Design review of the part built by this model. Coordinates are the model's own, in mm. Face numbers are marked on the shaded views. A direction names the side the tool comes from. Give positions to 0.01 mm unless a question says otherwise; leave off trailing zeros. Order: outer loops, then holes, each group sorted by start corner. A loop starts at its lowest first (then second) coordinate and runs counter-clockwise, first axis right, second up.
```python
from build123d import *

# Parameters (mm, degrees)
F0_W     = 10
F0_H     = 20
F1_DEPTH = 10
F2_W     = 7.14
F2_H     = 7
F3_DEPTH = 25
F4_DEPTH = 25
F5_DEPTH = 25


with BuildPart() as f1:
    # F0 (on Top) → F1 (new body)
    with BuildSketch(Plane.XY):
        with Locations((5, 10)):
            Rectangle(F0_W, F0_H)
    extrude(amount=F1_DEPTH)

    # F2 (on face) → F3 (cut)
    with BuildSketch(Plane.XY.offset(10)):
        with Locations((5, 15)):
            Rectangle(F2_W, F2_H)
    extrude(amount=-F3_DEPTH, mode=Mode.SUBTRACT)

    # F4 (add): a face of the model
    f4_faces = [f1.faces().sort_by_distance(p)[0] for p in [
        (5, 20, 5),
    ]]
    extrude(f4_faces, amount=F4_DEPTH)

    # F5 (add): a face of the model
    f5_faces = [f1.faces().sort_by_distance(p)[0] for p in [
        (5, 23.4370781461, 10),
    ]]
    extrude(f5_faces, amount=F5_DEPTH)


solid = f1.part
```
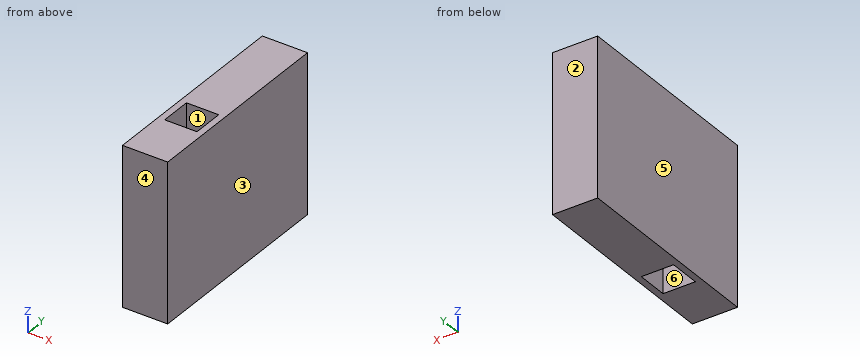
1. Take a section at C-C (x = 7.75). State the section outline as (y, z) points, then the cut area to 3 significant figures.
Recorded:
outline: (0, 0) - (11.5, 0) - (11.5, 35) - (0, 35) - close; (18.5, 0) - (45, 0) - (45, 35) - (18.5, 35) - close
area: 1,330 mm2
2. Take a section at A-A (y = 18). State the section outline as (x, z) points.
Recorded:
outline: (0, 0) - (1.43, 0) - (1.43, 35) - (0, 35) - close; (8.57, 0) - (10, 0) - (10, 35) - (8.57, 35) - close
3. For pin 1 (1 mm diameter, centred on x = 2.5, y = 13.5, fed in from +Z), flat-tipped, find the tip position at first contact; note if it passes through.
Recorded:
pin 1: passes through
4. Take a section at B-B (z = 32.5). State the section outline as (x, y) points.
Recorded:
outline: (0, 0) - (10, 0) - (10, 45) - (0, 45) - close; hole (1.43, 11.5) - (8.57, 11.5) - (8.57, 18.5) - (1.43, 18.5) - close
5. For line 1 along X through (y, z) = (15, 33); line 2 along Y through (x, z) = (8.5, 18), list the stretches that pass through material, from the lowest coordinate up.
Recorded:
line 1: x = 0 to 1.43, 8.57 to 10
line 2: y = 0 to 11.5, 18.5 to 45
6. Machinability: for the marked faces 1 and 2, which of the approach directions +Z, -Z, +X, -X, +Y, -Y give a long, thin tool a straight path to every point of the face, cutting with its end or side? Answer none if there is none.
Recorded:
face 1: +Z, -Z
face 2: +Z, -Z, +X, -X, +Y
7. Draft analysis for pull direction X (two halves, no side actions). For the marked faces 3, 4, 5 and 6, state which applies: pulls with the +X half, pulls with the -X half, needs draft (parallel to the pull), parting line crosses it, or undercut.
Recorded:
face 3: pulls with the +X half
face 4: needs draft
face 5: pulls with the -X half
face 6: undercut
